Input: part model. Units: mm. Frame: model coordinates. Face numbers are marked on the shaded views. A direction names the side the tool comes from. Round coordinates to 2 decimals unless told otherwise and drop trailing zeros. Loops run counter-clockwise (first coordinate to the right, second up) from the corner with the lowest first, then second, coordinate; pieces in that order, holes last.
(1) Draft query along X for the marked faces 1, 2 and 3. Return one class per face: released by +X, released by -X, zero draft, split by the parting line, or undercut.
(2) Cut plane D-D, the plane y = 49.5. Output: boundary loops of the cut face in (x, z), and give its area (3 significant figures).
(3) Cut plane A-A, the plane z = 122. Output: boundary loops of the cut face in (x, y), and give its area (3 significant figures).
(4) First-contact query: pin 1 Ø10 at (x, y) = (161, 93) entering from +Z; pin 2 Ø2 at (y, z) = (22, 114) entering from -X. Flat tips, straight axial feed; report the tip coordinate or a pass-through.
(5) Line query: line 1 (X direction, y = 56, z = 128.5); line 2 (X direction, y = 9.5, z = 26.5); line 3 (Y direction, x = 137, z = 28.5). Output: solid intervals per line, ascending.
(6) Cut plane C-C, the plane z = 15.5. Output: boundary loops of the cut face in (x, y), and give its area (4 significant figures).
(7) Access query for the marked faces 4, 5 and 6. Directions: +Z, -Z, +X, -X, +Y, -Y. A direction counts if a zero-diameter tool reaches every point of the face in a straight line with its end or side. Return the directions, or none.
(8) Cut plane B-B, the plane y = 64.5. Output: boundary loops of the cut face in (x, z).
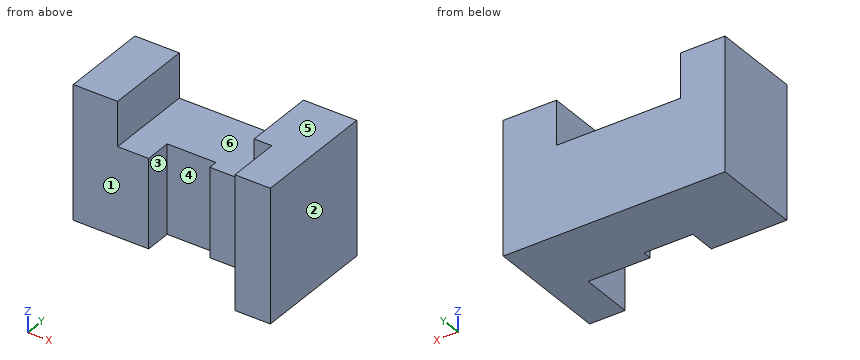
from build123d import *

# Parameters (mm, degrees)
F0_W     = 250
F0_H     = 150
F1_DEPTH = 140
F2_W     = 140
F2_H     = 50
F3_DEPTH = 140.001
F4_W     = 210
F4_H     = 40
F5_DEPTH = 150.001
F6_W     = 55
F6_H     = 30
F7_DEPTH = 100.001
F8_W     = 70
F8_H     = 20
F9_DEPTH = 150.001


with BuildPart() as f1:
    # F0 (on Front) → F1 (new body)
    with BuildSketch(Plane.XZ):
        with Locations((125, 75)):
            Rectangle(F0_W, F0_H)
    extrude(amount=-F1_DEPTH)

    # F2 (on face) → F3 (cut, through all)
    with BuildSketch(Plane.XZ):
        with Locations((120, 125)):
            Rectangle(F2_W, F2_H)
    extrude(amount=-F3_DEPTH, mode=Mode.SUBTRACT)

    # F4 (on face) → F5 (cut, through all)
    with BuildSketch(Plane(origin=(0, 0, 0), x_dir=(1, 0, 0), z_dir=(0, 0, -1))):
        with Locations((105, -20)):
            Rectangle(F4_W, F4_H)
    extrude(amount=-F5_DEPTH, mode=Mode.SUBTRACT)

    # F6 (on face) → F7 (cut, through all)
    with BuildSketch(Plane.XY.offset(100)):
        with Locations((112.5, 55)):
            Rectangle(F6_W, F6_H)
    extrude(amount=-F7_DEPTH, mode=Mode.SUBTRACT)

    # F8 (on face) → F9 (cut, through all)
    with BuildSketch(Plane(origin=(0, 0, 0), x_dir=(1, 0, 0), z_dir=(0, 0, -1))):
        with Locations((175, -50)):
            Rectangle(F8_W, F8_H)
    extrude(amount=-F9_DEPTH, mode=Mode.SUBTRACT)


solid = f1.part
Reported:
1. face 1: zero draft
1. face 2: released by +X
1. face 3: undercut
2. outline: (0, 0) - (85, 0) - (85, 100) - (50, 100) - (50, 150) - (0, 150) - close; (210, 0) - (250, 0) - (250, 150) - (210, 150) - close
2. area: 17,000 mm2
3. outline: (0, 40) - (50, 40) - (50, 140) - (0, 140) - close; (190, 60) - (210, 60) - (210, 0) - (250, 0) - (250, 140) - (190, 140) - close
3. area: 12,200 mm2
4. pin 1: stops at z = 100
4. pin 2: stops at x = 210
5. line 1: x = 0 to 50, 210 to 250
5. line 2: x = 210 to 250
5. line 3: y = 70 to 140
6. outline: (0, 40) - (85, 40) - (85, 70) - (140, 70) - (140, 60) - (210, 60) - (210, 0) - (250, 0) - (250, 140) - (0, 140) - close
6. area: 23,550 mm2
7. face 4: +Z, -Z, -Y
7. face 5: +Z, +X, -X, +Y, -Y
7. face 6: +Z, +Y, -Y
8. outline: (0, 0) - (85, 0) - (85, 100) - (50, 100) - (50, 150) - (0, 150) - close; (140, 0) - (250, 0) - (250, 150) - (190, 150) - (190, 100) - (140, 100) - close
